Source: three-view drawing plus pictorial views. Frame: mm from the lowest corner of the part. Give positions to 0.01 mm unless a question says otherwise; leave off trailing zeros. Write each loop counter-clockwise with the first axis right and the second up, starting at its lowest first coordinate (ties: lowest second). Pieces come first, ordered by that corner, then holes.
Q1. Line query: L1, parallel to Y at x = 45.5, z = 2.5. Output: solid intervals per line, ascending.
Q2. Cut plane A-A on z = 18. Return the cut outline in (x, y), plus the area to 3 significant figures.
Q3. Pin query (flat end, axial travel): pin 1 (1.6 mm diameter, centred on y = 71.5, z = 1, fed in from -X); pin 2 (22 mm diameter, centred on x = 108, y = 71.5, fed in from +Z). Return the tip coordinate at first contact, or that it passes through.
Q4. Cut plane C-C on y = 27.5. Return the cut outline in (x, z), plus the area to 3 significant figures.
Q5. Cut plane B-B on x = 67.5. Return the cut outline in (y, z).
Q6. Draft query along Y for the marked faces 1, 2, 3 and 4. Return one class per face: pulls with the +Y half, pulls with the -Y half, needs draft (parallel to the pull), parting line crosses it, or undercut.
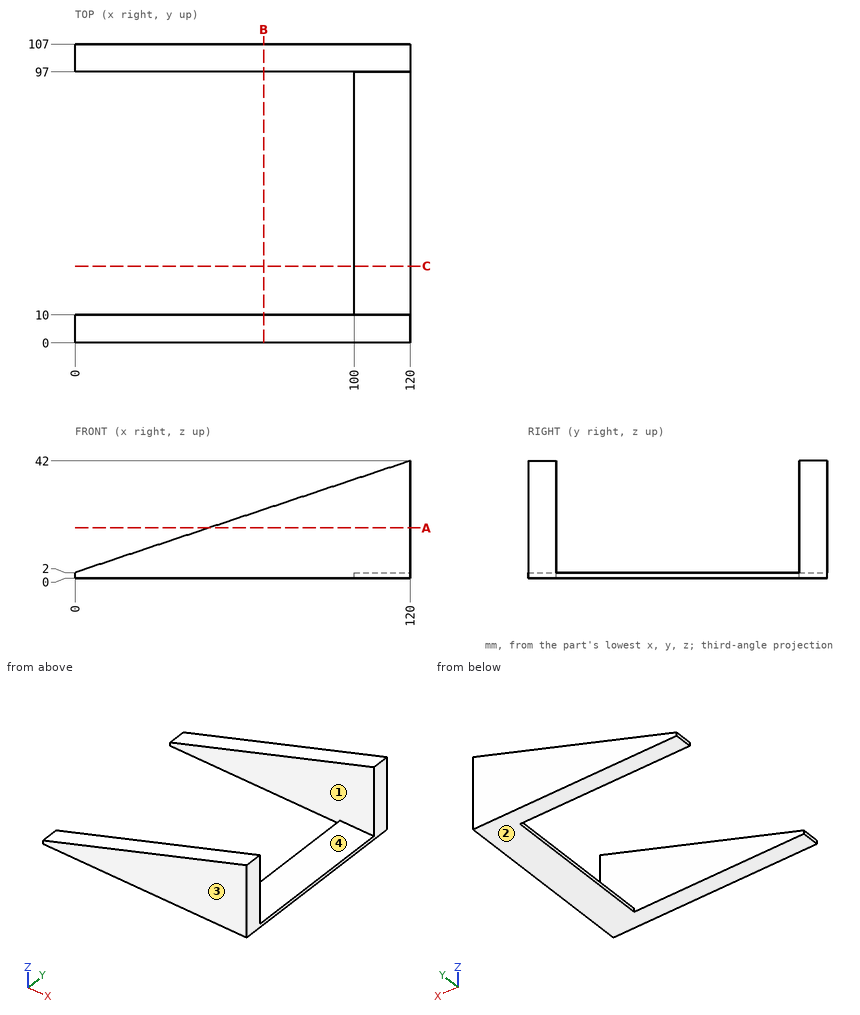
Data:
1. L1: y = 0 to 10, 97 to 107
2. outline: (48, 0) - (120, 0) - (120, 10) - (48, 10) - close; (48, 97) - (120, 97) - (120, 107) - (48, 107) - close
2. area: 1,440 mm2
3. pin 1: stops at x = 100
3. pin 2: stops at z = 2
4. outline: (100, 0) - (120, 0) - (120, 2) - (100, 2) - close
4. area: 40.0 mm2
5. outline: (0, 0) - (10, 0) - (10, 24.5) - (0, 24.5) - close; (97, 0) - (107, 0) - (107, 24.5) - (97, 24.5) - close
6. face 1: undercut
6. face 2: needs draft
6. face 3: pulls with the -Y half
6. face 4: undercut
